The listing builds one solid part. Answer for the finished solid, in the listing's coordinates (mm). A direction names the side the tool comes from. Coordinates: 2 decimals unless noted, no trailing zeros. Loops run counter-clockwise (first coordinate to the right, second up) from the corner with the lowest first, then second, coordinate; pieces in that order, holes last. Notation, with made-up numbers: (48, -20) - (76, -20) arc R15 cw to (76, 5) - close; hole circle Ø5 at (63, 11.25). An arc over 180 degrees is marked (long way). Return JSON: item names as keys, results as strings. Group by question number.
1. Section D-D (x = -87) is taken. Write down the section's boundary in (y, z) (3 decimals).
2. Each of these flat-tipped pins is pushed along its axis until it touches: P1, Ø1.9, axis at x = -46.5, z = -1, coming from the -Y side; P2, Ø10, axis at x = 0, y = 0, coming from the +Z side (3 decimals). Where does it stop, or does it pass through?
3. Find the intervals of material crossed by line 1 along Y through (x, z) = (-127, 0.5) (3 decimals); line 2 along X through (y, z) = (-2.25, 1.5); line 3 along Y through (x, z) = (-22, -2.75), in increasing order.
4. Which of the six approach directions +Z, -Z, +X, -X, +Y, -Y give full straight-line access (tool end or side, diameter ignored) to faces 1 (the face through (-119.46, -6.67, 0.04)), 2 (the face through (-0.69, -3.1, -0.04)), 3 (the face through (-64, 6.35, 0))?
5. Section C-C (z = -1.75) is taken. Write down the section's boundary in (x, y) (3 decimals), and give its area (3 significant figures).
6. The mould has two halves that part along X. Classify faces 4 (the face through (-7.54, 6.67, 0.04)), 5 (the face through (-62, 0, 3.175)): pulls with the +X half, pulls with the -X half, needs draft (parallel to the pull), parting line crosses it, or undercut.
7. Section B-B (x = -127) is taken. Write down the section's boundary in (y, z) (3 decimals).
8. Section A-A (y = 0) is taken. Write down the section's boundary in (x, z) (3 decimals), and give its area (3 significant figures).
```python
from build123d import *

# Parameters (mm, degrees)
SKETCH1_R           = 3.175
BOSS_EXTRUDE1_DEPTH = 3.175


with BuildPart() as part:
    # Sketch1 → Boss-Extrude1 (new, symmetric)
    with BuildSketch(Plane.XY):
        with BuildLine():
            Line((-117.475, 6.35), (-9.525, 6.35))
            ThreePointArc((-9.525, 6.35), (-7.516953686, 6.675861057), (-5.715, 7.62))
            ThreePointArc((-5.715, 7.62), (9.525, 0), (-5.715, -7.62))
            ThreePointArc((-5.715, -7.62), (-7.516953686, -6.675861057), (-9.525, -6.35))
            Line((-9.525, -6.35), (-117.475, -6.35))
            ThreePointArc((-117.475, -6.35), (-119.483046314, -6.675861057), (-121.285, -7.62))
            ThreePointArc((-121.285, -7.62), (-136.525, 0), (-121.285, 7.62))
            ThreePointArc((-121.285, 7.62), (-119.483046314, 6.675861057), (-117.475, 6.35))
        make_face()
        with Locations((-127, 0)):
            Circle(SKETCH1_R, mode=Mode.SUBTRACT)
        Circle(SKETCH1_R, mode=Mode.SUBTRACT)
    extrude(amount=BOSS_EXTRUDE1_DEPTH, both=True)


solid = part.part
```
The answers:
{
 "1": {"outline": "(-6.35, -3.175) - (6.35, -3.175) - (6.35, 3.175) - (-6.35, 3.175) - close"},
 "2": {"P1": "stops at y = -6.35", "P2": "stops at z = 3.175"},
 "3": {"line 1": "y = -9.525 to -3.175, 3.175 to 9.525", "line 2": "x = -136.26 to -129.24, -124.76 to -2.24, 2.24 to 9.26", "line 3": "y = -6.35 to 6.35"},
 "4": {"face 1": "+Z, -Z, -Y", "face 2": "+Z, -Z", "face 3": "+Z, -Z, +Y"},
 "5": {"outline": "(-121.285, -7.62) arc R6.35 cw to (-117.475, -6.35) - (-9.525, -6.35) arc R6.35 cw to (-5.715, -7.62) arc R9.525 ccw (long way) to (-5.715, 7.62) arc R6.35 cw to (-9.525, 6.35) - (-117.475, 6.35) arc R6.35 cw to (-121.285, 7.62) arc R9.525 ccw (long way) to start; hole circle Ø6.35 at (-127, 0); hole circle Ø6.35 at (0, 0)", "area": "1,900 mm2"},
 "6": {"face 4": "undercut", "face 5": "needs draft"},
 "7": {"outline": "(-9.525, -3.175) - (-3.175, -3.175) - (-3.175, 3.175) - (-9.525, 3.175) - close; (3.175, -3.175) - (9.525, -3.175) - (9.525, 3.175) - (3.175, 3.175) - close"},
 "8": {"outline": "(-136.525, -3.175) - (-130.175, -3.175) - (-130.175, 3.175) - (-136.525, 3.175) - close; (-123.825, -3.175) - (-3.175, -3.175) - (-3.175, 3.175) - (-123.825, 3.175) - close; (3.175, -3.175) - (9.525, -3.175) - (9.525, 3.175) - (3.175, 3.175) - close", "area": "847 mm2"}
}
